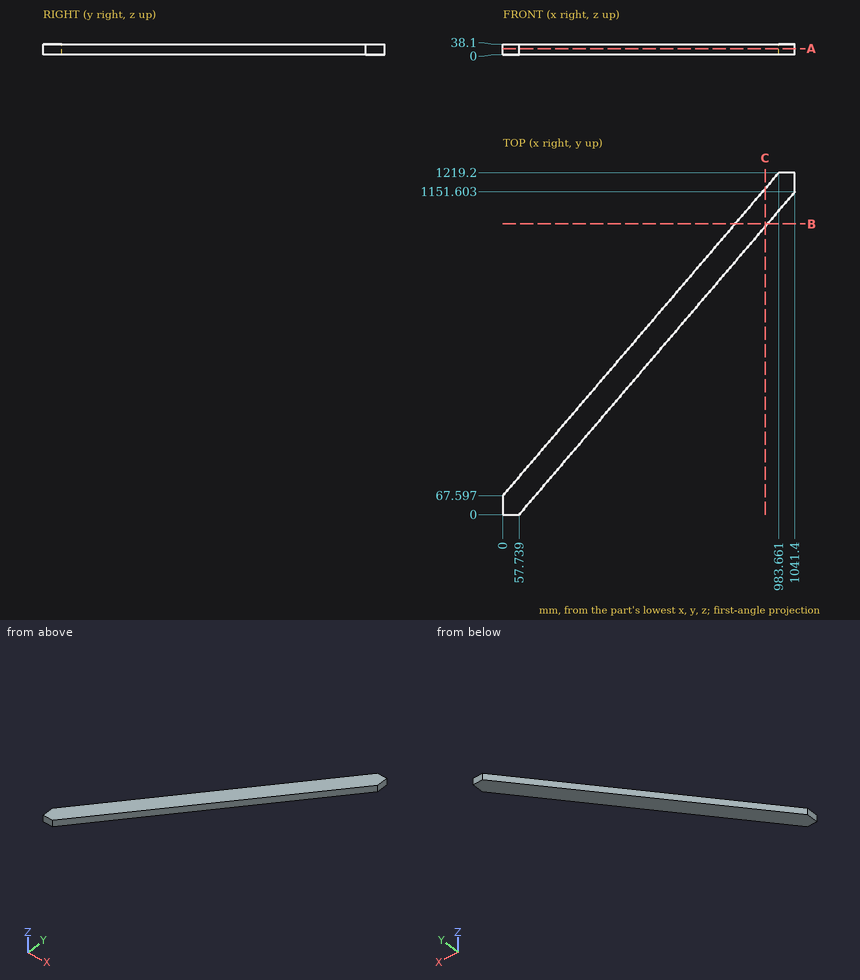
Could you check a few things on this drawing? It's one solid part, dimensions in mm from its lowest x, y, z. Coordinates: 2 decimals unless noted, no trailing zeros. Order: outer loops, then holes, each group sorted by start corner. A loop starts at its lowest first (then second) coordinate and runs counter-clockwise, first axis right, second up. Notation, with made-up numbers: (84, 45.25) -> (129, 45.25) arc R16 cw to (129, 51.25) -> close; hole circle Ø10 at (31.5, 58.5). An arc over 180 degrees is marked (long way). Answer in a Markdown table with one row per item.
(1) Please list where these lines run through material, in increasing order: probe 1 along Y at (x, z) = (368, 6.5) (1 decimal); probe 2 along Y at (x, z) = (757.5, 35.5) (1 decimal); probe 3 along X at (y, z) = (251, 27.5) (1 decimal).
Answer key:
| item | result |
|---|---|
| probe 1 | 363.2 to 498.4 |
| probe 2 | 819.2 to 954.4 |
| probe 3 | 156.7 to 272.1 |
(2) I want a section at A-A on z = 22. List the corners of the cut face in (x, y) for me.
Answer key:
| item | result |
|---|---|
| outline | (0, 0) -> (57.74, 0) -> (1041.4, 1151.6) -> (1041.4, 1219.2) -> (983.66, 1219.2) -> (0, 67.6) -> close |
(3) I want a section at C-C on x = 935. List the corners of the cut face in (y, z) for me.
Answer key:
| item | result |
|---|---|
| outline | (1027.04, 0) -> (1162.23, 0) -> (1162.23, 38.1) -> (1027.04, 38.1) -> close |
(4) I want a section at B-B on y = 1037. List the corners of the cut face in (x, z) for me, then the cut area to 3 significant figures.
Answer key:
| item | result |
|---|---|
| outline | (828.03, 0) -> (943.51, 0) -> (943.51, 38.1) -> (828.03, 38.1) -> close |
| area | 4,400 mm^2 |
(5) Will these pins go through, and if not, where does the flat tip stop? pin 1 Ø10 at (x, z) = (425, 21.5) entering from +Y; pin 2 Ø6 at (x, z) = (377.5, 16) entering from +Y; pin 3 Ø10 at (x, z) = (860.5, 16) entering from -Y (1 decimal).
Answer key:
| item | result |
|---|---|
| pin 1 | y = 571.01 |
| pin 2 | y = 513.06 |
| pin 3 | y = 934 |
